Design review of the part built by this model. Coordinates are the model's own, in mm. A direction names the side the tool comes from. Round coordinates to 2 decimals unless told otherwise and drop trailing zeros. Loops run counter-clockwise (first coordinate to the right, second up) from the corner with the lowest first, then second, coordinate; pieces in that order, holes last. Notation, with made-up numbers: M -28.75,82.5 L -10.75,82.5 A30 cw -10.75,112.5 Z; hole C 73,17.5 d10. An arc over 180 degrees is marked long. Answer as CSV lines item,"result". Start each with the question number.
from build123d import *

# Parameters (mm, degrees)
F0_W     = 88.9
F0_H     = 88.9
F1_DEPTH = 6.35
F2_W     = 88.9
F2_H     = 88.9
F2_W_2   = 81.28
F2_H_2   = 81.28
F3_DEPTH = 12.7
F4_R     = 6.35
F5_DEPTH = 6.351


with BuildPart() as f1:
    # F0 (on Top) → F1 (new body)
    with BuildSketch(Plane.XY):
        with Locations((44.45, 44.45)):
            Rectangle(F0_W, F0_H)
    extrude(amount=F1_DEPTH)

    # F2 (on face) → F3 (join)
    with BuildSketch(Plane.XY.offset(6.35)):
        with Locations((44.45, 44.45)):
            Rectangle(F2_W, F2_H)
        with Locations((44.45, 44.45)):
            Rectangle(F2_W_2, F2_H_2, mode=Mode.SUBTRACT)
    extrude(amount=F3_DEPTH)

    # F4 (on face) → F5 (cut, through all)
    with BuildSketch(Plane.XY.offset(6.35)):
        with Locations((17.280384, 71.619616)):
            Circle(F4_R)
        with Locations((17.280384, 17.280384)):
            Circle(F4_R)
        with Locations((71.619616, 17.280384)):
            Circle(F4_R)
        with Locations((71.619616, 71.619616)):
            Circle(F4_R)
    extrude(amount=-F5_DEPTH, mode=Mode.SUBTRACT)


solid = f1.part
Item 1: Insertion check: pin 1 Ø16.5 at (x, y) = (71.62, 17.28) entering from +Z; pin 2 Ø10 at (x, y) = (71.62, 71.62) entering from +Z. Each pin has a flat end and moves straight along its axis. Give the tip position at first contact, or say it passes through.
Item 2: Consider section B-B, the plane x = 67. Write out the cut boundary in (y, z), then the cut area to 3 significant figures.
Item 3: The part is to be moulded in two halves that separate along Y. For faces 3 (the face through (88.9, 44, 9)), 4 (the face through (44, 0, 9)), 5 (the face through (70.24, 65.42, 3.22)), say which applies: +Y half, -Y half, draft (parallel to the pull), parting line (faces both ways), or undercut.
Item 4: Tool access review of faces 1 (the face through (15.9, 65.42, 3.22)), 2 (the face through (44, 45, 6.35)): name each direction out of +Z, -Z, +X, -X, +Y, -Y from which nothing blocks a thin tool from reaching the whole face with its end or side.
Item 5: To check wall thickness, follow line 1 (X direction, y = 28.5, z = 8); line 2 (Y direction, x = 72, z = 5.5). State the ranges of each line that lie inside material, in increasing order.
Item 6: Consider section C-C, the plane y = 15. Write out the cut boundary in (x, z).
Item 7: Consider section D-D, the plane y = 45. Write out the cut boundary in (x, z).
Item 8: Consider section A-A, the plane z = 17. Write out the cut boundary in (x, y).
Found:
1,pin 1,"stops at z = 6.35"
1,pin 2,"passes through"
2,outline,"M 0,0 L 12.92,0 L 12.92,6.35 L 3.81,6.35 L 3.81,19.05 L 0,19.05 Z; M 21.64,0 L 67.26,0 L 67.26,6.35 L 21.64,6.35 Z; M 75.98,0 L 88.9,0 L 88.9,19.05 L 85.09,19.05 L 85.09,6.35 L 75.98,6.35 Z"
2,area,"551 mm^2"
3,face 3,"draft"
3,face 4,"-Y half"
3,face 5,"undercut"
4,face 1,"+Z, -Z"
4,face 2,"+Z"
5,line 1,"x = 0 to 3.81, 85.09 to 88.9"
5,line 2,"y = 0 to 10.94, 23.62 to 65.28, 77.96 to 88.9"
6,outline,"M 0,0 L 11.35,0 L 11.35,6.35 L 3.81,6.35 L 3.81,19.05 L 0,19.05 Z; M 23.21,0 L 65.69,0 L 65.69,6.35 L 23.21,6.35 Z; M 77.55,0 L 88.9,0 L 88.9,19.05 L 85.09,19.05 L 85.09,6.35 L 77.55,6.35 Z"
7,outline,"M 0,0 L 88.9,0 L 88.9,19.05 L 85.09,19.05 L 85.09,6.35 L 3.81,6.35 L 3.81,19.05 L 0,19.05 Z"
8,outline,"M 0,0 L 88.9,0 L 88.9,88.9 L 0,88.9 Z; hole M 3.81,3.81 L 85.09,3.81 L 85.09,85.09 L 3.81,85.09 Z"
